The listing builds one solid part. Answer for the finished solid, in the listing's coordinates (mm). Face numbers are marked on the shaded views. A direction names the side the tool comes from. Coordinates: 2 decimals unless noted, no trailing zeros. Order: outer loops, then holes, each group sorted by start corner. A loop starts at its lowest first (then second) coordinate and runs counter-clockwise, first axis right, second up.
from build123d import *

# Parameters (mm, degrees)
SKETCH2_R           = 4.997903731
SKETCH2_R_2         = 2.1
BOSS_EXTRUDE1_DEPTH = 2


with BuildPart() as part:
    # Sketch1 → Revolve2 (revolve)
    with BuildSketch(Plane.XY, mode=Mode.PRIVATE) as revolve2_sk:
        with BuildLine():
            Line((0, 2.1), (8.384411392, 2.1))
            Line((8.384411392, 2.1), (21, 2.1))
            Line((21, 2.1), (21, 2.592))
            ThreePointArc((21, 2.592), (20.851210245, 2.951210245), (20.492, 3.1))
            Line((20.492, 3.1), (20, 3.1))
            Line((20, 3.1), (14, 4.485209147))
            Line((14, 4.485209147), (14, 3.1))
            Line((14, 3.1), (0, 3.1))
            Line((0, 3.1), (0, 2.1))
        make_face()
    revolve(revolve2_sk.sketch.rotate(Axis((0, 0, 0), (1, 0, 0)), 90), axis=Axis((0, 0, 0), (1, 0, 0)))

    # Sketch2 → Boss-Extrude1 (add)
    with BuildSketch(Plane.ZY):
        Circle(SKETCH2_R)
        Circle(SKETCH2_R_2, mode=Mode.SUBTRACT)
    extrude(amount=BOSS_EXTRUDE1_DEPTH)


solid = part.part
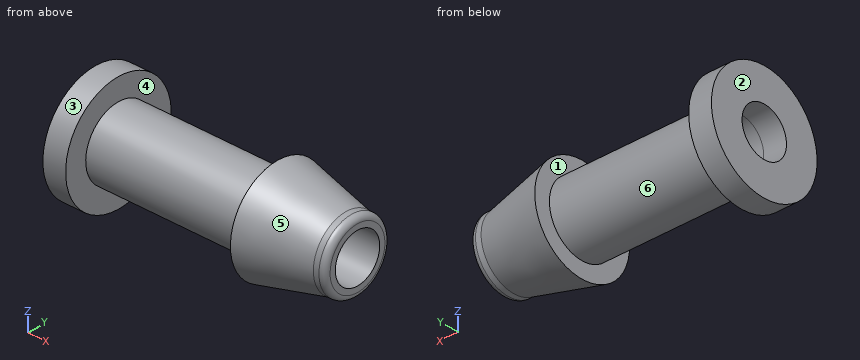
(1) The mould has two halves that part along X. Classify the marked faces 1, 2, 3 and 4: pulls with the +X half, pulls with the -X half, needs draft (parallel to the pull), parting line crosses it, or undercut.
(2) Given pin 1 Ø3 at (x, z) = (11.5, -1.5) entering from +Y; pin 2 Ø5 at (x, z) = (14, -2.5) entering from -Y; pin 3 Ø3 at (x, z) = (0.5, 3.5) entering from +Y, each flat-ended and moving along its own axis, determine where each tip first touches the part or whether it passes through.
(3) Find the intervals of material crossed by probe 1 along Y at (x, z) = (8.75, 0); probe 2 along Y at (x, z) = (-0.75, 0); probe 3 along Z at (x, y) = (12, 0.75), in increasing order.
(4) A tool of negligible diameter and unlimited length cuts with its end or side. For the marked faces 5 and 6, from which of +Z, -Z, +X, -X, +Y, -Y can it reach the whole face along a straight path? Write none if from no direction.
(5) Find section A-A on z = 0. Determine the outline of the cut face in (x, y).
(6) Find section D-D on x = -0.5. Determine the outline of the cut face in (y, z).
(7) Find section C-C on x = 4.75. Determine the outline of the cut face in (y, z), then the cut area to 3 significant figures.
Resolved:
1. face 1: undercut
1. face 2: pulls with the -X half
1. face 3: needs draft
1. face 4: undercut
2. pin 1: stops at y = 3.1
2. pin 2: stops at y = -4.49
2. pin 3: stops at y = 4.54
3. probe 1: y = -3.1 to -2.1, 2.1 to 3.1
3. probe 2: y = -5 to -2.1, 2.1 to 5
3. probe 3: z = -3.01 to -1.96, 1.96 to 3.01
4. face 5: +X
4. face 6: none
5. outline: (-2, -5) - (0, -5) - (0, -3.1) - (14, -3.1) - (14, -4.49) - (20, -3.1) - (20.49, -3.1) arc R0.51 ccw to (21, -2.59) - (21, -2.1) - (-2, -2.1) - close; (-2, 2.1) - (21, 2.1) - (21, 2.59) arc R0.51 ccw to (20.49, 3.1) - (20, 3.1) - (14, 4.49) - (14, 3.1) - (0, 3.1) - (0, 5) - (-2, 5) - close
6. outline: circle Ø10 at (0, 0); hole circle Ø4.2 at (0, 0)
7. outline: circle Ø6.2 at (0, 0); hole circle Ø4.2 at (0, 0)
7. area: 16.3 mm2
